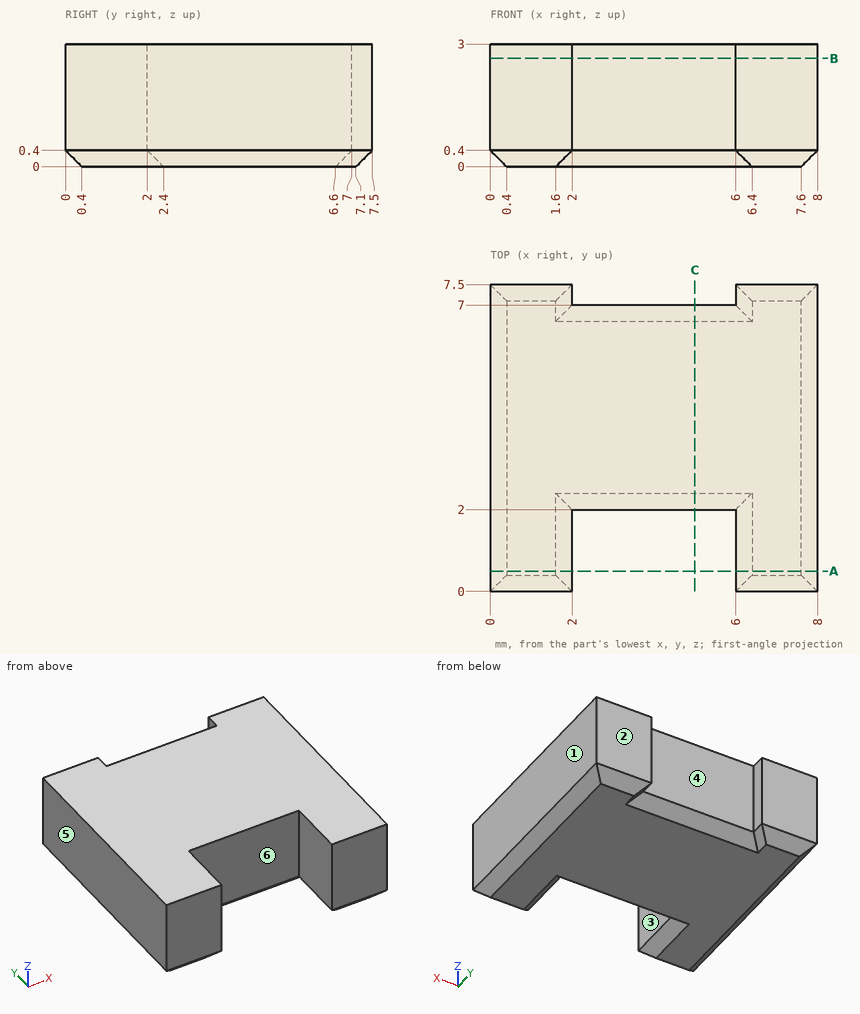
The drawing under review shows one solid part. Ordinate dimensions are in mm from its lowest x, y, z. A direction names the side the tool comes from. Give positions to 0.01 mm unless a question says otherwise; leave off trailing zeros. Write each loop counter-clockwise with the first axis right and the second up, starting at its lowest first coordinate (ties: lowest second). Pieces come first, ordered by that corner, then holes. Notation, with made-up numbers: (-16.75, 1.25) - (-4.75, 1.25) arc R20 cw to (-4.75, 40.25) - close; hole circle Ø3 at (-38, -37.75). An arc over 180 degrees is marked (long way). Answer in a Markdown table with one row per item. Add a question column.
1. Draft analysis for pull direction X (two halves, no side actions). For the marked faces 1, 2 and 3, state which applies: +X half, -X half, draft (parallel to the pull), parting line (faces both ways), or undercut.
2. Wall thickness on line 1 along X through (y, z) = (1.75, 0.7); line 2 along Y through (x, z) = (4, 1.75); line 3 along Y through (x, z) = (6.5, 0.35): over which ranges is each line inside the solid? List them lowest first. Write a range as [from, to].
3. We need section B-B on z = 2.65. Write out the cut boundary in (x, y).
4. We need section A-A on y = 0.5. Write out the cut boundary in (x, z).
5. We need section C-C on x = 5. Write out the cut boundary in (y, z), then the cut area to 3 significant figures.
6. Tool access review of the marked faces 4, 5 and 6: name each direction out of +Z, -Z, +X, -X, +Y, -Y from which nothing blocks a thin tool from reaching the whole face with its end or side.
7. Insertion check: P1, Ø1.5, axis at x = 4, y = 1.5, coming from the -Z side. The pin has a flat end and moves straight along its axis. Give the tip position at first contact, or say it passes through.
Ans:
| question | item | result |
|---|---|---|
| 1 | face 1 | +X half |
| 1 | face 2 | draft |
| 1 | face 3 | undercut |
| 2 | line 1 | x = [0, 2], [6, 8] |
| 2 | line 2 | y = [2, 7] |
| 2 | line 3 | y = [0.05, 7.45] |
| 3 | outline | (0, 0) - (2, 0) - (2, 2) - (6, 2) - (6, 0) - (8, 0) - (8, 7.5) - (6, 7.5) - (6, 7) - (2, 7) - (2, 7.5) - (0, 7.5) - close |
| 4 | outline | (0, 0.4) - (0.4, 0) - (1.6, 0) - (2, 0.4) - (2, 3) - (0, 3) - close; (6, 0.4) - (6.4, 0) - (7.6, 0) - (8, 0.4) - (8, 3) - (6, 3) - close |
| 5 | outline | (2, 0.4) - (2.4, 0) - (6.6, 0) - (7, 0.4) - (7, 3) - (2, 3) - close |
| 5 | area | 14.8 mm^2 |
| 6 | face 4 | +Z, -Z, +Y |
| 6 | face 5 | +Z, -Z, -X, +Y, -Y |
| 6 | face 6 | +Z, -Z, -Y |
| 7 | P1 | stops at z = 0.15 |
